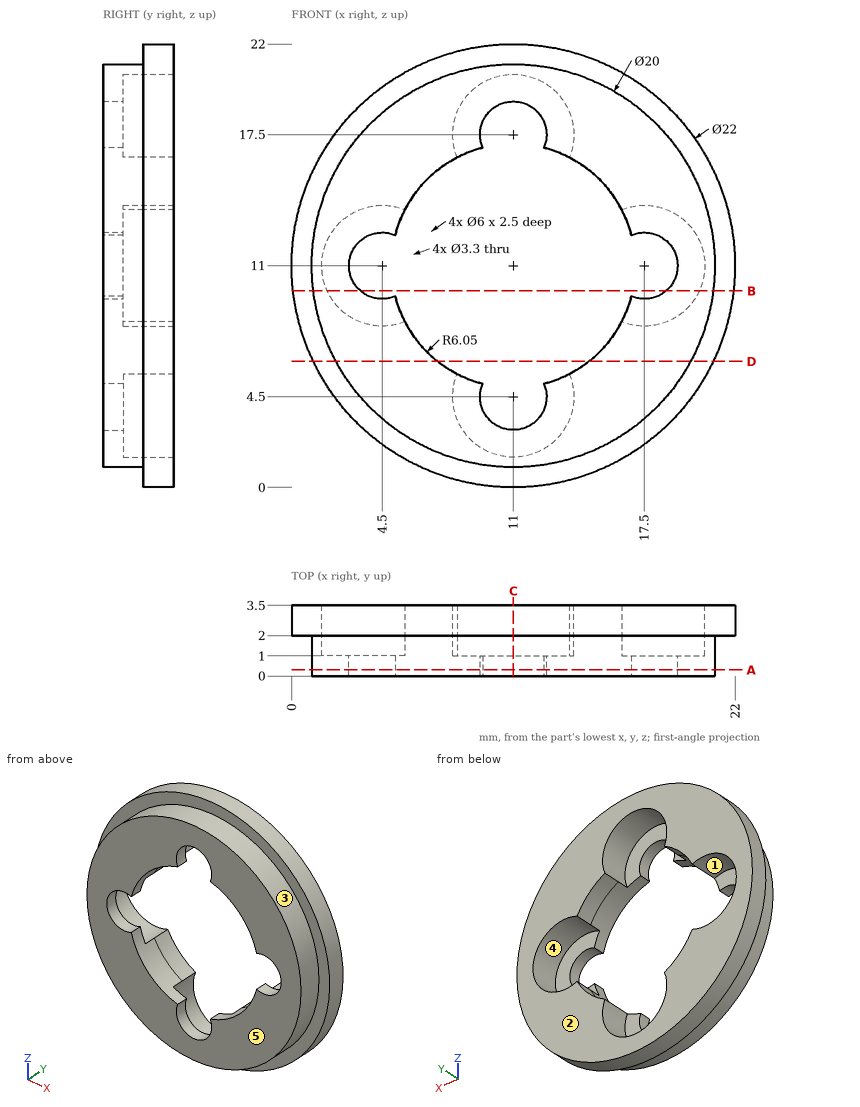
Geometry: see drawing. Coordinates: mm, zero at the bounding-box minimum. A direction names the side the tool comes from. Coordinates: 2 decimals unless noted, no trailing zeros. Loops run counter-clockwise (first coordinate to the right, second up) from the corner with the lowest first, then second, coordinate; pieces in that order, holes last.
Q1. Draft query along Z for the marked faces 1, 2 and 3. Return one class per face: +Z half, -Z half, draft (parallel to the pull), parting line (faces both ways), or undercut.
Q2. Material intervals for line 1 (X direction, y = 2.7, z = 11); line 2 (Z direction, x = 14, y = 0.35); line 3 (Z direction, x = 15, y = 2.8), sorted ascending.
Q3. Cut plane D-D (z = 6.25). Output: boundary loops of the cut face in (x, y), then the cut area to 3 significant figures.
Q4. Cut plane A-A (y = 0.3). Output: boundary loops of the cut face in (x, z), then the cut area to 3 significant figures.
Q5. Cut plane C-C (x = 11). Output: boundary loops of the cut face in (y, z), then the cut area to 3 significant figures.
Q6. Set-up query: the marked faces 4 and 5. Return all of +Z, -Z, +X, -X, +Y, -Y with unobstructed straight access to the full face (end or side cutting, diameter ignored); none if empty.
Q7. Cut plane B-B (z = 9.75). Output: boundary loops of the cut face in (x, y), then the cut area to 3 significant figures.
Q8. Contact query for flat-ended pins moving along their axis: pin 1 (1.2 mm diameter, centred on x = 18.5, z = 9.5, fed in from +Y); pin 2 (2 mm diameter, centred on y = 2.5, z = 7, fed in from +X). Output: stop coordinate, or through.
Working result:
1. face 1: undercut
1. face 2: draft
1. face 3: parting line
2. line 1: x = 0 to 1.5, 20.5 to 22
2. line 2: z = 1.46 to 5.75, 16.25 to 20.54
2. line 3: z = 0.75 to 6.46, 15.54 to 21.25
3. outline: (1.08, 2) - (2.2, 2) - (2.2, 0) - (7.25, 0) - (7.25, 3.5) - (1.08, 3.5) - close; (14.75, 0) - (19.8, 0) - (19.8, 2) - (20.92, 2) - (20.92, 3.5) - (14.75, 3.5) - close
3. area: 38.7 mm2
4. outline: circle Ø20 at (11, 11); hole (5.14, 9.48) arc R6.05 ccw to (9.48, 5.14) arc R1.65 ccw (long way) to (12.52, 5.14) arc R6.05 ccw to (16.86, 9.48) arc R1.65 ccw (long way) to (16.86, 12.52) arc R6.05 ccw to (12.52, 16.86) arc R1.65 ccw (long way) to (9.48, 16.86) arc R6.05 ccw to (5.14, 12.52) arc R1.65 ccw (long way) to start
4. area: 175 mm2
5. outline: (0, 1) - (2, 1) - (2, 0) - (3.5, 0) - (3.5, 1.5) - (1, 1.5) - (1, 2.85) - (0, 2.85) - close; (0, 19.15) - (1, 19.15) - (1, 20.5) - (3.5, 20.5) - (3.5, 22) - (2, 22) - (2, 21) - (0, 21) - close
5. area: 9.20 mm2
6. face 4: +Y
6. face 5: +Z, -Z, +X, -X, -Y
7. outline: (0.07, 2) - (1.08, 2) - (1.08, 0) - (3.42, 0) - (3.42, 1) - (1.77, 1) - (1.77, 3.5) - (0.07, 3.5) - close; (18.58, 0) - (20.92, 0) - (20.92, 2) - (21.93, 2) - (21.93, 3.5) - (20.23, 3.5) - (20.23, 1) - (18.58, 1) - close
7. area: 11.2 mm2
8. pin 1: stops at y = 1
8. pin 2: stops at x = 21.58
